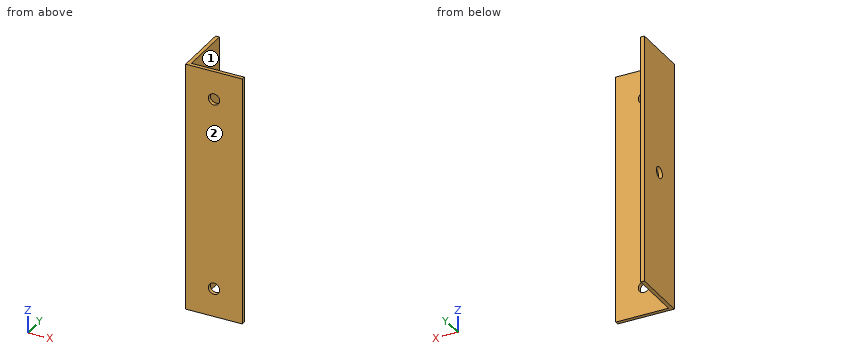
from build123d import *

# Parameters (mm, degrees)
EXTRUDE_1_DEPTH     = 66
SKETCH_3_R          = 1.5
CUT_EXTRUDE_1_DEPTH = 10
SKETCH_4_R          = 1.5
CUT_EXTRUDE_2_DEPTH = 10
SKETCH_5_R          = 1.5
CUT_EXTRUDE_3_DEPTH = 10


with BuildPart() as part:
    # ｽｹｯﾁ1 → ﾎﾞｽ - 押し出し1 (new body)
    with BuildSketch(Plane.XY):
        Polygon((-4.461455774, 6.353305785), (-5.461455774, 6.353305785), (-5.461455774, -8.646694215), (9.538544226, -8.646694215), (9.538544226, -7.646694215), (-4.461455774, -7.646694215), align=None)
    extrude(amount=EXTRUDE_1_DEPTH)

    # ｽｹｯﾁ3 → ｶｯﾄ - 押し出し1 (cut)
    with BuildSketch(Plane(origin=(-4.461455774, 0, 0), x_dir=(0, 0, -1), z_dir=(1, 0, 0))):
        with Locations((-33, -1.146694215)):
            Circle(SKETCH_3_R)
    extrude(amount=-CUT_EXTRUDE_1_DEPTH, mode=Mode.SUBTRACT)

    # ｽｹｯﾁ4 → ｶｯﾄ - 押し出し2 (cut)
    with BuildSketch(Plane(origin=(0, -7.646694215, 0), x_dir=(1, 0, 0), z_dir=(0, 1, 0))):
        with Locations((2.038544226, -7.5)):
            Circle(SKETCH_4_R)
    extrude(amount=-CUT_EXTRUDE_2_DEPTH, mode=Mode.SUBTRACT)

    # ｽｹｯﾁ5 → ｶｯﾄ - 押し出し3 (cut)
    with BuildSketch(Plane(origin=(0, -7.646694215, 0), x_dir=(1, 0, 0), z_dir=(0, 1, 0))):
        with Locations((2.038544226, -58.5)):
            Circle(SKETCH_5_R)
    extrude(amount=-CUT_EXTRUDE_3_DEPTH, mode=Mode.SUBTRACT)


solid = part.part
The listing builds one solid part. Answer for the finished solid, in the listing's coordinates (mm). Face numbers are marked on the shaded views. A direction names the side the tool comes from. Coordinates: 2 decimals unless noted, no trailing zeros. Write each loop counter-clockwise with the first axis right and the second up, starting at its lowest first coordinate (ties: lowest second). Pieces come first, ordered by that corner, then holes. Notation, with made-up numbers: (51.25, 20.25) - (98.25, 20.25) arc R18 cw to (98.25, 52.25) - close; hole circle Ø8 at (-3.5, 24). An arc over 180 degrees is marked (long way). Put each result on its own line as item: value.
1. Find the intervals of material crossed by line 1 along X through (y, z) = (-8.4, 7.5); line 2 along Y through (x, z) = (-5, 33); line 3 along X through (y, z) = (-1, 7), in increasing order. Write a range as from..to.
Answer sheet:
line 1: x = -5.46..0.54, 3.54..9.54
line 2: y = -8.65..-2.65, 0.35..6.35
line 3: x = -5.46..-4.46
2. The part is cut by section A-A on z = 7.5. Give the vertices of the cut face in (x, y).
Answer sheet:
outline: (-5.46, -8.65) - (0.54, -8.65) - (0.54, -7.65) - (-4.46, -7.65) - (-4.46, 6.35) - (-5.46, 6.35) - close; (3.54, -8.65) - (9.54, -8.65) - (9.54, -7.65) - (3.54, -7.65) - close
3. The part is cut by section B-B on y = -5.25. Give the vertices of the cut face in (x, z).
Answer sheet:
outline: (-5.46, 0) - (-4.46, 0) - (-4.46, 66) - (-5.46, 66) - close
4. The part is cut by section D-D on z = 16.5. Give the vertices of the cut face in (x, y).
Answer sheet:
outline: (-5.46, -8.65) - (9.54, -8.65) - (9.54, -7.65) - (-4.46, -7.65) - (-4.46, 6.35) - (-5.46, 6.35) - close
5. Flat-ended cylindrical pins translate along their axes: pin 1 Ø7 at (x, z) = (4, 33.5) entering from +Y; pin 2 Ø4 at (y, z) = (-1.15, 33) entering from +X; pin 3 Ø3 at (x, y) = (-1.5, 3) entering from +Z. Find the tip coordinate at first contact, or state that the pin passes through.
Answer sheet:
pin 1: stops at y = -7.65
pin 2: stops at x = -4.46
pin 3: passes through
6. A tool of negligible diameter and unlimited length cuts with its end or side. For the marked faces 1 and 2, from which of +Z, -Z, +X, -X, +Y, -Y can it reach the whole face along a straight path? Write none if from no direction.
Answer sheet:
face 1: +Z, -Z, +X, +Y
face 2: +Z, -Z, +X, -X, -Y
7. The part is cut by section C-C on x = -2.25. Give the vertices of the cut face in (y, z).
Answer sheet:
outline: (-8.65, 0) - (-7.65, 0) - (-7.65, 66) - (-8.65, 66) - close
